Geometry: final body of the model. Coordinates: model frame, mm. Face numbers are marked on the shaded views. A direction names the side the tool comes from. Give positions to 0.01 mm unless a question says otherwise; leave off trailing zeros. Loops run counter-clockwise (first coordinate to the right, second up) from the corner with the lowest first, then second, coordinate; pieces in that order, holes last. Notation, with made-up numbers: (28.5, -19) -> (65.5, -19) arc R34 cw to (65.5, 20) -> close; hole circle Ø1 at (33, -6). An arc over 180 degrees is marked (long way). Answer in a Markdown table with one row per item. Add a question column.
1) Section query D-D (x = 73). Return the cut outline in (y, z).
2) Section query B-B (z = -28). Return the cut outline in (x, y).
3) Section query A-A (y = 8). Return the cut outline in (x, z).
4) Access query for the marked faces 1, 2 and 3. Directions: +Z, -Z, +X, -X, +Y, -Y. A direction counts if a zero-diameter tool reaches every point of the face in a straight line with its end or side. Return the directions, or none.
5) Section query C-C (x = 16). Return the cut outline in (y, z), plus the area to 3 significant figures.
6) Line query: line 1 (Z direction, x = 75.5, y = 8); line 2 (Z direction, x = 63, y = 5.75); line 3 (Y direction, x = 72.5, z = -31). Output: solid intervals per line, ascending. Write a range as from..to.
7) Draft query along X for the marked faces 4, 5 and 6. Return one class per face: +X half, -X half, draft (parallel to the pull), parting line (faces both ways), or undercut.
8) First-contact query: P1, Ø1.5, axis at x = 20, y = 5, coming from the +Z side; P2, Ø4, axis at x = 39, z = 18.5, coming from the +Y side; P3, Ø4, axis at y = 7.5, z = 16.5, coming from the +X side; P4, Ø1, axis at x = 13, z = -16, coming from the +Y side. Flat tips, straight axial feed; report the tip coordinate or a pass-through.
```python
from build123d import *

# Parameters (mm, degrees)
BOSS_EXTRUDE1_DEPTH = 1.5
SKETCH2_W           = 58.5
SKETCH2_H           = 5
BOSS_EXTRUDE2_DEPTH = 8
SKETCH3_W           = 10
SKETCH3_H           = 10
BOSS_EXTRUDE3_DEPTH = 8
SKETCH4_R           = 5
BOSS_EXTRUDE4_DEPTH = 12


with BuildPart() as part:
    # Sketch1 → Boss-Extrude1 (new body)
    with BuildSketch(Plane(origin=(0, 0, 0), x_dir=(1, 0, 0), z_dir=(0, 1, 0))):
        Polygon((0, 0), (0, -21.5), (90, -21.5), (90, 33.5), (6, 33.5), (6, 18), (20, 18), (20, 0), align=None)
    extrude(amount=BOSS_EXTRUDE1_DEPTH)

    # Sketch2 → Boss-Extrude2 (add)
    with BuildSketch(Plane(origin=(0, 1.5, 0), x_dir=(1, 0, 0), z_dir=(0, 1, 0))):
        with Locations((48.25, -17.5)):
            Rectangle(SKETCH2_W, SKETCH2_H)
        with Locations((48.25, 29.5)):
            Rectangle(SKETCH2_W, SKETCH2_H)
    extrude(amount=BOSS_EXTRUDE2_DEPTH)

    # Sketch3 → Boss-Extrude3 (add)
    with BuildSketch(Plane(origin=(0, 1.5, 0), x_dir=(1, 0, 0), z_dir=(0, 1, 0))):
        with Locations((55, 18)):
            Rectangle(SKETCH3_W, SKETCH3_H)
        with Locations((55, 5.912448656)):
            Rectangle(SKETCH3_W, SKETCH3_H)
        with Locations((55, -6)):
            Rectangle(SKETCH3_W, SKETCH3_H)
    extrude(amount=BOSS_EXTRUDE3_DEPTH)

    # Sketch4 → Boss-Extrude4 (add)
    with BuildSketch(Plane(origin=(0, 1.5, 0), x_dir=(1, 0, 0), z_dir=(0, 1, 0))):
        with Locations(Location((67, 18, 0), (0, 0, 270))):
            Circle(SKETCH4_R)
        with Locations(Location((67, 5.912448656, 0), (0, 0, 270))):
            Circle(SKETCH4_R)
        with Locations(Location((67, -6, 0), (0, 0, 270))):
            Circle(SKETCH4_R)
    extrude(amount=BOSS_EXTRUDE4_DEPTH)


solid = part.part
```
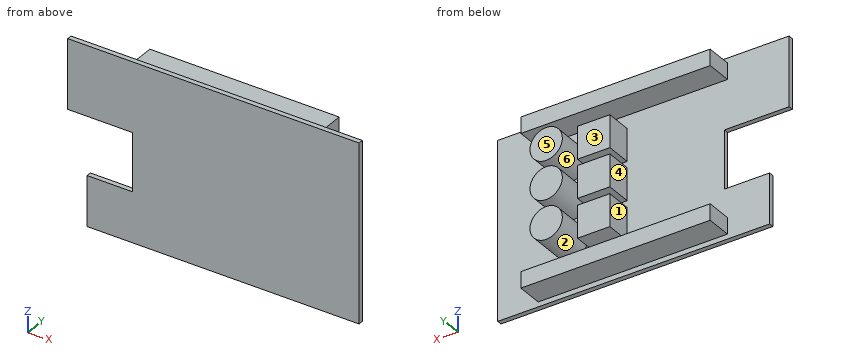
Evaluation:
| question | item | result |
|---|---|---|
| 1 | outline | (0, -33.5) -> (1.5, -33.5) -> (1.5, -32) -> (9.5, -32) -> (9.5, -27) -> (1.5, -27) -> (1.5, 15) -> (9.5, 15) -> (9.5, 20) -> (1.5, 20) -> (1.5, 21.5) -> (0, 21.5) -> close |
| 2 | outline | (6, 0) -> (90, 0) -> (90, 1.5) -> (77.5, 1.5) -> (77.5, 9.5) -> (19, 9.5) -> (19, 1.5) -> (6, 1.5) -> close |
| 3 | outline | (19, -32) -> (77.5, -32) -> (77.5, -27) -> (19, -27) -> close; (19, 15) -> (77.5, 15) -> (77.5, 20) -> (19, 20) -> close; (50, -23) -> (60, -23) -> (60, -13) -> (50, -13) -> close; (50, -10.91) -> (60, -10.91) -> (60, -0.91) -> (50, -0.91) -> close; (50, 1) -> (60, 1) -> (60, 11) -> (50, 11) -> close; circle Ø10 at (67, -18); circle Ø10 at (67, -5.91); circle Ø10 at (67, 6) |
| 4 | face 1 | -X, +Y |
| 4 | face 2 | +Y |
| 4 | face 3 | +Z, -Z, -X, +Y |
| 5 | outline | (0, -33.5) -> (1.5, -33.5) -> (1.5, -18) -> (0, -18) -> close; (0, 0) -> (1.5, 0) -> (1.5, 21.5) -> (0, 21.5) -> close |
| 5 | area | 55.5 mm² |
| 6 | line 1 | -32..-27, 15..20 |
| 6 | line 2 | -32..-27, -21..-15, -8.91..-2.91, 3..9, 15..20 |
| 6 | line 3 | 0..9.5 |
| 7 | face 4 | -X half |
| 7 | face 5 | draft |
| 7 | face 6 | undercut |
| 8 | P1 | z = 20 |
| 8 | P2 | y = 9.5 |
| 8 | P3 | x = 77.5 |
| 8 | P4 | through |
